CAD build for the part. Positions are in the model's coordinates, mm. A direction names the side the tool comes from. Give positions to 0.01 mm unless a question says otherwise; leave off trailing zeros. Order: outer loops, then holes, each group sorted by start corner. A loop starts at its lowest first (then second) coordinate and runs counter-clockwise, first axis right, second up.
Autodesk Inventor part; units mm, degrees
ref_plane "YZ Plane" through (0, 0, 0) normal (1, 0, 0) x (0, 1, 0)
ref_plane "XZ Plane" through (0, 0, 0) normal (0, 1, 0) x (-1, 0, 0)
ref_plane "XY Plane" through (0, 0, 0) normal (0, 0, 1) x (1, 0, 0)
sketch "Эскиз1" plane through (0, 0, 0) normal (0, 1, 0) x (-1, 0, 0)
  circle A0 centre (0, 0) radius 40
  dimension "d0" = 80
extrude "Выдавливание1" add sketch "Эскиз1" along normal blind 25
sketch "Эскиз2" plane through (0, 25, 0) normal (0, 1, 0) x (1, 0, 0)
  circle A0 centre (0, 0) radius 24
  dimension "d3" = 48
extrude "Выдавливание2" cut sketch "Эскиз2" against normal blind 6
sketch "Эскиз3" plane through (0, 19, 0) normal (0, 1, 0) x (1, 0, 0)
  circle A0 centre (0, 0) radius 16
  dimension "d6" = 32
extrude "Выдавливание3" cut sketch "Эскиз3" against normal blind 55.25
sketch "Эскиз4" plane through (0, 0, 0) normal (0, -1, 0) x (1, 0, 0)
  circle A0 centre (0, 0) radius 22
  dimension "d9" = 44
extrude "Выдавливание4" cut sketch "Эскиз4" against normal blind 9
chamfer "Фаска1" distance 1.6 angle 45 1 edges at (-22, 0, 0)
sketch "Эскиз5" plane through (0, 0, 0) normal (0, -1, 0) x (1, 0, 0)
  point P0 (0, 0)
  point P1 (0, 30)
  point P2 (0, -30)
  dimension "d15" = 30
  dimension "d16" = 30
hole "Отверстие1" at (0, 0, 30) at (0, 0, -30) direction (0, 1, 0) diameter 6.647 depth 15.5 tip angle 118
chamfer "Фаска2" distance 1.6 angle 45 1 edges at (0, 0, 33.3235)
chamfer "Фаска3" distance 1.6 angle 45 1 edges at (0, 0, -26.6765)
properties part number "Корпус"
1. Saw through at D-D on x = 33. Give the cut face in (y, z).
2. Saw through at C-C on y = 10.25. Give the cut face in (x, z).
3. Saw through at B-B on y = 5.25. Give the cut face in (x, z).
4. Mould opens along Z. For faces 4 (the flat face through (-17, 0, -17)), 5 (the cylindrical face through (8.67, 12.32, 39.05)), 6 (the flat face through (1.5, 9, -16.2)) say: released by +Z, released by -Z, zero draft, split by the parting line, or undercut.
5. Wall check: line 1 (Z direction, x = 0, y = 11.25); line 2 (Z direction, x = 0, y = 4.75); line 3 (Z direction, x = 0, y = 22.45). Give the ranges that are in metal, low to high.
6. Saw through at A-A on z = 0. Give the cut face in (x, y), plus the area to 3 significant figures.
7. 3-axis set-ups, long thin cutter, end or side, ignore diameter. For faces 1 (the cylindrical face through (-3.47, 14.07, 15.62)), 2 (the cylindrical face through (-23.977, 22.042, -1.055)), 3 (the cylindrical face through (2.02, 8.65, -27.36)): which of +Z, -Z, +X, -X, +Y, -Y reach the whole face in a straight line?
8. Pin check, flat tips, straight feed: P1, Ø1.5, axis at x = 10, z = 15, coming from the -Y side; P2, Ø2, axis at y = 22, z = 4, coming from the +X side; P3, Ø10, axis at y = 22.5, z = -6, coming from the -X side; P4, Ø2, axis at x = 31.5, z = -29, coming from the +Y side. Stop position of each tip, or through.
Reported:
1. outline: (0, -22.61) - (25, -22.61) - (25, 22.61) - (0, 22.61) - close
2. outline: circle Ø80 at (0, 0); hole circle Ø32 at (0, 0); hole circle Ø6.65 at (0, -30); hole circle Ø6.65 at (0, 30)
3. outline: circle Ø80 at (0, 0); hole circle Ø44 at (0, 0); hole circle Ø6.65 at (0, -30); hole circle Ø6.65 at (0, 30)
4. face 4: zero draft
4. face 5: split by the parting line
4. face 6: undercut
5. line 1: z = -40 to -33.32, -26.68 to -16, 16 to 26.68, 33.32 to 40
5. line 2: z = -40 to -33.32, -26.68 to -22, 22 to 26.68, 33.32 to 40
5. line 3: z = -40 to -24, 24 to 40
6. outline: (-40, 0) - (-23.6, 0) - (-22, 1.6) - (-22, 9) - (-16, 9) - (-16, 19) - (-24, 19) - (-24, 25) - (-40, 25) - close; (16, 9) - (22, 9) - (22, 1.6) - (23.6, 0) - (40, 0) - (40, 25) - (24, 25) - (24, 19) - (16, 19) - close
6. area: 993 mm2
7. face 1: +Y, -Y
7. face 2: +Y
7. face 3: -Y
8. P1: stops at y = 9
8. P2: stops at x = 39.89
8. P3: stops at x = -39.99
8. P4: passes through
